from build123d import *

# Parameters (mm, degrees)
CUT_EXTRUDE_7_DEPTH      = 187.681547026
CUT_EXTRUDE_7_DEPTH_BACK = 187.681547026
SKETCH_10_W              = 30
SKETCH_10_H              = 10
SKETCH_14_R              = 8
CUT_EXTRUDE_8_DEPTH      = 191.065778087
SKETCH_6_W               = 18
SKETCH_6_H               = 4
CUT_EXTRUDE_4_DEPTH      = 4
CHAMFER_3_SIZE           = 2
CHAMFER_4_SIZE           = 4


with BuildPart() as part:
    # Эскиз1 → Повернуть1 (revolve)
    with BuildSketch(Plane.XY, mode=Mode.PRIVATE) as revolve_1_sk:
        Polygon((0, 0), (0, 25), (80, 25), (80, 35), (120, 35), (120, 15), (180, 15), (180, 0), align=None)
    revolve(revolve_1_sk.sketch.rotate(Axis((0, 0, 0), (-1, 0, 0)), 90), axis=Axis((0, 0, 0), (-1, 0, 0)))

    # Эскиз10 → Вырез-Вытянуть7 (cut, two sides: drawn at the far end of the back side and taken through both)
    with BuildSketch(Plane.XY.offset(-CUT_EXTRUDE_7_DEPTH_BACK)):
        with Locations((55, 20)):
            Rectangle(SKETCH_10_W, SKETCH_10_H)
    extrude(amount=CUT_EXTRUDE_7_DEPTH + CUT_EXTRUDE_7_DEPTH_BACK, mode=Mode.SUBTRACT)

    # Эскиз14 → Вырез-Вытянуть8 (cut, through all)
    with BuildSketch(Plane(origin=(0, 15, 0), x_dir=(1, 0, 0), z_dir=(0, 1, 0))):
        with Locations(Location((55, 0, 0), (0, 0, 270))):
            Circle(SKETCH_14_R)
    extrude(amount=-CUT_EXTRUDE_8_DEPTH, mode=Mode.SUBTRACT)

    # Эскиз6 → Вырез-Вытянуть4 (cut, symmetric)
    with BuildSketch(Plane.XY):
        with Locations((146, 13)):
            Rectangle(SKETCH_6_W, SKETCH_6_H)
    extrude(amount=CUT_EXTRUDE_4_DEPTH, both=True, mode=Mode.SUBTRACT)

    # Фаска3
    chamfer_3_edges = [part.edges().sort_by_distance(p)[0] for p in [
        (180, 0, 15),
    ]]
    chamfer(chamfer_3_edges, length=CHAMFER_3_SIZE)

    # Фаска4
    chamfer_4_edges = [part.edges().sort_by_distance(p)[0] for p in [
        (0, 0, 25),
    ]]
    chamfer(chamfer_4_edges, length=CHAMFER_4_SIZE)


solid = part.part
The listing builds one solid part. Answer for the finished solid, in the listing's coordinates (mm). A direction names the side the tool comes from. Give positions to 0.01 mm unless a question says otherwise; leave off trailing zeros. Loops run counter-clockwise (first coordinate to the right, second up) from the corner with the lowest first, then second, coordinate; pieces in that order, holes last. Notation, with made-up numbers: (65, 20) - (85, 20) arc R12 cw to (85, 27) - close; hole circle Ø9 at (52.5, 35). An arc over 180 degrees is marked (long way). Answer as a JSON object with one key per item and string values.
1. Find the intervals of material crossed by L1, parallel to Z at x = 55, y = -15; L2, parallel to X at y = -6, z = 0; L3, parallel to Y at x = 169, z = 1, in increasing order. Write a range as [from, to].
Determined:
{"L1": "[-20, -8], [8, 20]", "L2": "[0, 47], [63, 180]", "L3": "[-14.97, 14.97]"}
2. A cutting plane is placed at A-A (z = 0). Write down the section's boundary in (x, y), then the cut area to 3 significant figures.
Determined:
{"outline": "(0, -21) - (4, -25) - (47, -25) - (47, 15) - (40, 15) - (40, 25) - (4, 25) - (0, 21) - close; (63, -25) - (80, -25) - (80, -35) - (120, -35) - (120, -15) - (178, -15) - (180, -13) - (180, 13) - (178, 15) - (155, 15) - (155, 11) - (137, 11) - (137, 15) - (120, 15) - (120, 35) - (80, 35) - (80, 25) - (70, 25) - (70, 15) - (63, 15) - close", "area": "7,570 mm²"}
3. For a pull along X with two mould halves and no side action, classify faces 1 (the flat face through (180, 0, 0)), 2 (the flat face through (0, 0, 0)), 3 (the flat face through (146, 13, -4)) as pulls with the +X half, pulls with the -X half, needs draft (parallel to the pull), parting line crosses it, or undercut.
Determined:
{"face 1": "pulls with the +X half", "face 2": "pulls with the -X half", "face 3": "undercut"}
4. A cutting plane is placed at C-C (x = 49.5). Write down the section's boundary in (y, z).
Determined:
{"outline": "(-24.32, -5.81) arc R25 ccw to (15, -20) - (15, -5.81) - close; (-24.32, 5.81) - (15, 5.81) - (15, 20) arc R25 ccw to start"}
5. A cutting plane is placed at D-D (x = 132). Write down the section's boundary in (y, z), then the cut area to 3 significant figures.
Determined:
{"outline": "circle Ø30 at (0, 0)", "area": "707 mm²"}
6. A cutting plane is placed at B-B (y = 0). Write down the section's boundary in (x, z), then the cut area to 3 significant figures.
Determined:
{"outline": "(0, -21) - (4, -25) - (80, -25) - (80, -35) - (120, -35) - (120, -15) - (178, -15) - (180, -13) - (180, 13) - (178, 15) - (120, 15) - (120, 35) - (80, 35) - (80, 25) - (4, 25) - (0, 21) - close; hole circle Ø16 at (55, 0)", "area": "8,380 mm²"}
7. Flat-ended cylindrical pins translate along their axes: pin 1 Ø3 at (y, z) = (-25, 4.5) entering from -X; pin 2 Ø10 at (y, z) = (-17, -25) entering from -X; pin 3 Ø21 at (x, z) = (55, 0) entering from +Y. Find the tip coordinate at first contact, or state that the pin passes through.
Determined:
{"pin 1": "x = 2.9", "pin 2": "x = 80", "pin 3": "y = 15"}
8. For faces 4 (the cylindrical face through (149.41, -12.65, -8.06)), 5 (the flat face through (70, 19, 0)), 6 (the flat face through (146, 11, 0)), 7 (the flat face through (80, -8, -24)), determine the directions among +Z, -Z, +X, -X, +Y, -Y from which every point of the face is accessible in a straight line to the end or side of a thin tool.
Determined:
{"face 4": "+X", "face 5": "+Z, -Z, +Y", "face 6": "+Y", "face 7": "-X"}
